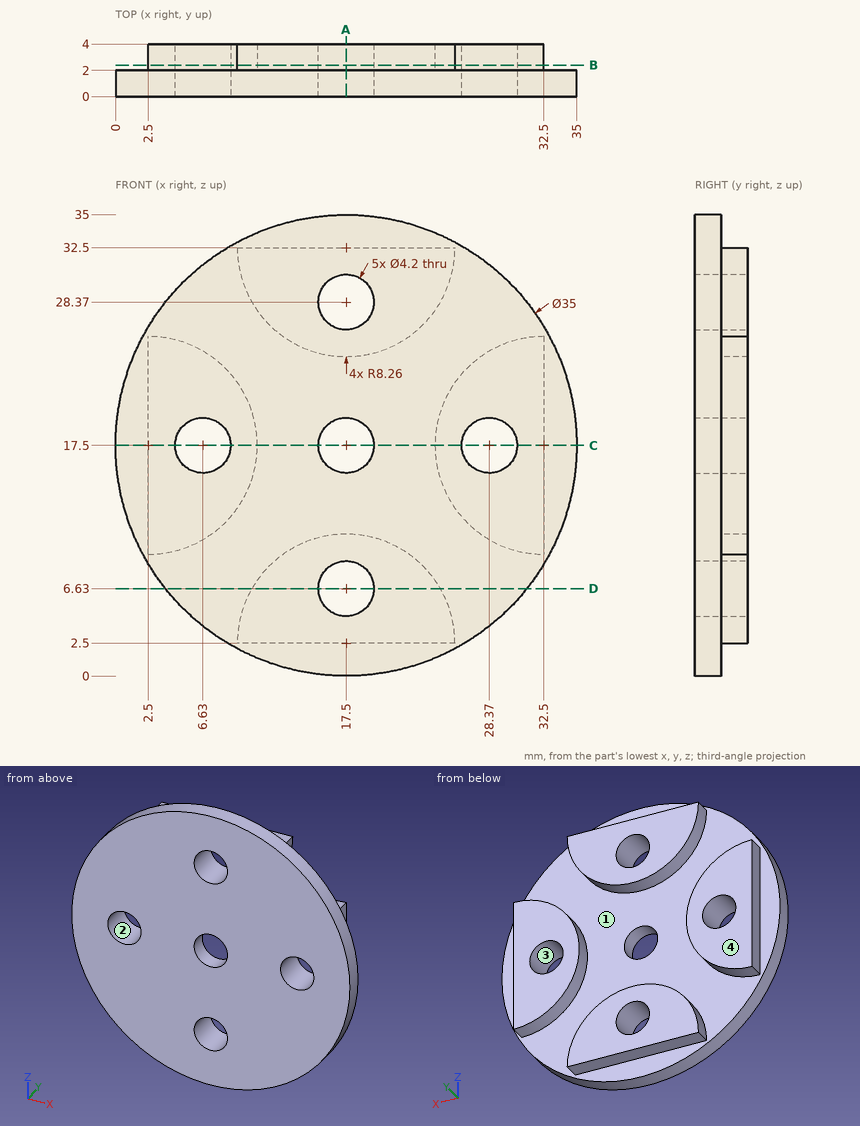
Can you work these out from the drawing? Everything is in mm from the part's minimum corner. A direction names the side the tool comes from. Round coordinates to 2 decimals unless told otherwise and drop trailing zeros. Write each loop counter-clockwise with the first axis right and the second up, starting at its lowest first coordinate (ties: lowest second). Pieces come first, ordered by that corner, then holes.
1. Suppose I cut it at D-D (z = 6.63). List the corners of the cut face in (x, y) for me, and give its area (3 significant figures).
2. If we mould it in two halves opening along Z, with no side actions, what happens to the marked faces 3 and 4? For each: released by +Z, released by -Z, zero draft, split by the parting line, or undercut.
3. For the marked faces 1 and 2, which set-ups out of +Z, -Z, +X, -X, +Y, -Y let a thin tool reach every point of the face, with its end or its side?
4. Suppose I cut it at B-B (y = 2.4). List the corners of the cut face in (x, z) for me, and give its area (3 significant figures).
5. Suppose I cut it at A-A (x = 17.5). List the corners of the cut face in (y, z) for me, and give its area (3 significant figures).
6. I need wall thicknesses on L1, parallel to Z at x = 17.5, y = 2.8; L2, parallel to Z at x = 17.5, y = 1.55. Which ranges of each line are inside material? Lowest first, please.
7. Suppose I cut it at C-C (z = 17.5). List the corners of the cut face in (x, y) for me.
8. Will these pins go through, and if not, where does the flat tip stop? pin 1 Ø0.6 at (x, y) = (19.5, 3.5) entering from +Z; pin 2 Ø1.5 at (y, z) = (2.5, 10.5) entering from -X; pin 3 Ø12 at (x, z) = (26, 30.5) entering from +Y; pin 4 Ø2 at (y, z) = (3.5, 16.5) entering from -X.
Answer sheet:
1. outline: (3.79, 0) - (15.4, 0) - (15.4, 4) - (10.35, 4) - (10.35, 2) - (3.79, 2) - close; (19.6, 0) - (31.21, 0) - (31.21, 2) - (24.65, 2) - (24.65, 4) - (19.6, 4) - close
1. area: 66.7 mm2
2. face 3: undercut
2. face 4: zero draft
3. face 1: +Y
3. face 2: +Y, -Y
4. outline: (2.5, 9.24) arc R8.26 ccw to (2.5, 25.76) - close; (9.24, 2.5) - (25.76, 2.5) arc R8.26 ccw to start; (9.24, 32.5) arc R8.26 ccw to (25.76, 32.5) - close; (32.5, 9.24) - (32.5, 25.76) arc R8.26 ccw to start; hole circle Ø4.2 at (6.63, 17.5); hole circle Ø4.2 at (17.5, 6.63); hole circle Ø4.2 at (17.5, 28.37); hole circle Ø4.2 at (28.37, 17.5)
4. area: 373 mm2
5. outline: (0, 0) - (2, 0) - (2, 2.5) - (4, 2.5) - (4, 4.53) - (0, 4.53) - close; (0, 8.73) - (4, 8.73) - (4, 10.76) - (2, 10.76) - (2, 15.4) - (0, 15.4) - close; (0, 19.6) - (2, 19.6) - (2, 24.24) - (4, 24.24) - (4, 26.27) - (0, 26.27) - close; (0, 30.47) - (4, 30.47) - (4, 32.5) - (2, 32.5) - (2, 35) - (0, 35) - close
5. area: 61.0 mm2
6. L1: z = 2.5 to 4.53, 8.73 to 10.76, 24.24 to 26.27, 30.47 to 32.5
6. L2: z = 0 to 4.53, 8.73 to 15.4, 19.6 to 26.27, 30.47 to 35
7. outline: (0, 0) - (4.53, 0) - (4.53, 4) - (2.5, 4) - (2.5, 2) - (0, 2) - close; (8.73, 0) - (15.4, 0) - (15.4, 2) - (10.76, 2) - (10.76, 4) - (8.73, 4) - close; (19.6, 0) - (26.27, 0) - (26.27, 4) - (24.24, 4) - (24.24, 2) - (19.6, 2) - close; (30.47, 0) - (35, 0) - (35, 2) - (32.5, 2) - (32.5, 4) - (30.47, 4) - close
8. pin 1: stops at z = 32.5
8. pin 2: stops at x = 1.23
8. pin 3: stops at y = 4
8. pin 4: stops at x = 2.5
